from build123d import *

# Parameters (mm, degrees)
SKETCH_1_W          = 23
SKETCH_1_H          = 23
EXTRUDE_1_DEPTH     = 1.6
SKETCH_2_W          = 5
SKETCH_2_H          = 4
EXTRUDE_2_DEPTH     = 1.6
FILLET_1_R          = 4
CUT_EXTRUDE_1_REACH = 18.575
SKETCH_3_R          = 1.6
CUT_EXTRUDE_2_REACH = 18.575
SKETCH_4_R          = 1.5


with BuildPart() as part:
    # 草图1 → 凸台-拉伸1 (new body)
    with BuildSketch(Plane(origin=(0, 0, 0), x_dir=(1, 0, 0), z_dir=(0, 1, 0))):
        Rectangle(SKETCH_1_W, SKETCH_1_H)
    extrude(amount=EXTRUDE_1_DEPTH)

    # 草图2 → 凸台-拉伸2 (add)
    with BuildSketch(Plane(origin=(0, 1.6, 0), x_dir=(1, 0, 0), z_dir=(0, 1, 0))):
        Rectangle(SKETCH_2_W, SKETCH_2_H)
    extrude(amount=EXTRUDE_2_DEPTH)

    # 圆角1
    fillet_1_edges = [part.edges().sort_by_distance(p)[0] for p in [
        (11.5, 0.8, 11.5),
        (-11.5, 0.8, 11.5),
        (-11.5, 0.8, -11.5),
        (11.5, 0.8, -11.5),
    ]]
    fillet(fillet_1_edges, radius=FILLET_1_R)

    # 草图3 → 切除-拉伸1 (cut, up to next)
    with BuildSketch(Plane.XZ, mode=Mode.PRIVATE) as cut_extrude_1_sk1:
        with Locations(Location((-8, 8, 0), (0, 0, 270))):
            Circle(SKETCH_3_R)
    cut_extrude_1_tool1 = extrude(cut_extrude_1_sk1.sketch, amount=-CUT_EXTRUDE_1_REACH, mode=Mode.PRIVATE) & part.part
    # 草图3 → 切除-拉伸1 (cut, up to next)
    with BuildSketch(Plane.XZ, mode=Mode.PRIVATE) as cut_extrude_1_sk2:
        with Locations(Location((8, 8, 0), (0, 0, 270))):
            Circle(SKETCH_3_R)
    cut_extrude_1_tool2 = extrude(cut_extrude_1_sk2.sketch, amount=-CUT_EXTRUDE_1_REACH, mode=Mode.PRIVATE) & part.part
    # 草图3 → 切除-拉伸1 (cut, up to next)
    with BuildSketch(Plane.XZ, mode=Mode.PRIVATE) as cut_extrude_1_sk3:
        with Locations(Location((8, -8, 0), (0, 0, 270))):
            Circle(SKETCH_3_R)
    cut_extrude_1_tool3 = extrude(cut_extrude_1_sk3.sketch, amount=-CUT_EXTRUDE_1_REACH, mode=Mode.PRIVATE) & part.part
    # 草图3 → 切除-拉伸1 (cut, up to next)
    with BuildSketch(Plane.XZ, mode=Mode.PRIVATE) as cut_extrude_1_sk4:
        with Locations(Location((-8, -8, 0), (0, 0, 270))):
            Circle(SKETCH_3_R)
    cut_extrude_1_tool4 = extrude(cut_extrude_1_sk4.sketch, amount=-CUT_EXTRUDE_1_REACH, mode=Mode.PRIVATE) & part.part
    add(cut_extrude_1_tool1.solids().sort_by_distance((-8, 0, 8))[0], mode=Mode.SUBTRACT)
    add(cut_extrude_1_tool2.solids().sort_by_distance((8, 0, 8))[0], mode=Mode.SUBTRACT)
    add(cut_extrude_1_tool3.solids().sort_by_distance((8, 0, -8))[0], mode=Mode.SUBTRACT)
    add(cut_extrude_1_tool4.solids().sort_by_distance((-8, 0, -8))[0], mode=Mode.SUBTRACT)

    # 草图4 → 切除-拉伸2 (cut, up to next)
    with BuildSketch(Plane.XZ, mode=Mode.PRIVATE) as cut_extrude_2_sk1:
        with Locations(Location((0, 0, 0), (0, 0, 270))):
            Circle(SKETCH_4_R)
    cut_extrude_2_tool1 = extrude(cut_extrude_2_sk1.sketch, amount=-CUT_EXTRUDE_2_REACH, mode=Mode.PRIVATE) & part.part
    add(cut_extrude_2_tool1.solids().sort_by_distance((0, 0, 0))[0], mode=Mode.SUBTRACT)


solid = part.part
The listing builds one solid part. Answer for the finished solid, in the listing's coordinates (mm). A direction names the side the tool comes from. Coordinates: 2 decimals unless noted, no trailing zeros. Write each loop counter-clockwise with the first axis right and the second up, starting at its lowest first coordinate (ties: lowest second). Pieces come first, ordered by that corner, then holes. Notation, with made-up numbers: M 33.25,14 L 64.25,14 A17 cw 64.25,35 Z; hole C 57,-5.5 d1. An arc over 180 degrees is marked long. Write each question's results on one line, items separated by ' | '.
Item 1: For a pull along Z with two mould halves and no side action, classify faces 1 (the face through (7.03, 0.79, 9.27)), 2 (the face through (0, 1, -11.5)), 3 (the face through (-8.97, 0.79, -6.73)), 4 (the face through (-0.2, 1.6, 2.4)) as released by +Z, released by -Z, zero draft, split by the parting line, or undercut.
Answer below:
face 1: undercut | face 2: released by -Z | face 3: undercut | face 4: zero draft
Item 2: Consider probe 1 along X at (y, z) = (1, 0); probe 2 along X at (y, z) = (0.95, -6.75); probe 3 along Z at (x, y) = (7, 0.85). Determine where each line is inside the solid, lowest interval first. Write a range as [from, to].
Answer below:
probe 1: [-11.5, -1.5], [1.5, 11.5] | probe 2: [-11.5, -9], [-7, 7], [9, 11.5] | probe 3: [-11.5, -9.25], [-6.75, 6.75], [9.25, 11.5]
Item 3: The part is cut by section A-A on z = 0. Determine the outline of the cut face in (x, y).
Answer below:
outline: M -11.5,0 L -1.5,0 L -1.5,3.2 L -2.5,3.2 L -2.5,1.6 L -11.5,1.6 Z; M 1.5,0 L 11.5,0 L 11.5,1.6 L 2.5,1.6 L 2.5,3.2 L 1.5,3.2 Z
Item 4: Which of the six approach directions +Z, -Z, +X, -X, +Y, -Y give full straight-line access (tool end or side, diameter ignored) to faces 5 (the face through (0, 0, 2)), 6 (the face through (0, 2, 2)), 7 (the face through (-2.5, 2, 0)), 8 (the face through (2.5, 2, 0)), 9 (the face through (-10.359, 0.811, -10.297))?
Answer below:
face 5: +Z, -Z, +X, -X, -Y | face 6: +Z, +X, -X, +Y | face 7: +Z, -Z, -X, +Y | face 8: +Z, -Z, +X, +Y | face 9: -Z, -X, +Y, -Y
Item 5: The part is cut by section C-C on x = 0. Determine the outline of the cut face in (y, z), and give its area (3 significant figures).
Answer below:
outline: M 0,-11.5 L 1.6,-11.5 L 1.6,-2 L 3.2,-2 L 3.2,-1.5 L 0,-1.5 Z; M 0,1.5 L 3.2,1.5 L 3.2,2 L 1.6,2 L 1.6,11.5 L 0,11.5 Z | area: 33.6 mm2
Item 6: The part is cut by section D-D on z = 8. Determine the outline of the cut face in (x, y).
Answer below:
outline: M -11.47,0 L -9.6,0 L -9.6,1.6 L -11.47,1.6 Z; M -6.4,0 L 6.4,0 L 6.4,1.6 L -6.4,1.6 Z; M 9.6,0 L 11.47,0 L 11.47,1.6 L 9.6,1.6 Z
Item 7: Given P1, Ø1.5, axis at x = -7, y = 2.5, coming from the -Z side; P2, Ø1.3, axis at y = 2.5, z = 0, coming from the +X side; P3, Ø5, axis at x = 8, z = 8, coming from the +Y side; P4, Ø0.8, axis at x = 0, y = 2.5, coming from the -Z side, each flat-ended and moving along its own axis, determine where each tip first touches the part or whether it passes through.
Answer below:
P1: through | P2: x = 2.5 | P3: y = 1.6 | P4: z = -2
Item 8: The part is cut by section B-B on y = 0.45. Determine the outline of the cut face in (x, z).
Answer below:
outline: M -11.5,-7.5 A4 ccw -7.5,-11.5 L 7.5,-11.5 A4 ccw 11.5,-7.5 L 11.5,7.5 A4 ccw 7.5,11.5 L -7.5,11.5 A4 ccw -11.5,7.5 Z; hole C -8,-8 d3.2; hole C -8,8 d3.2; hole C 0,0 d3; hole C 8,-8 d3.2; hole C 8,8 d3.2
